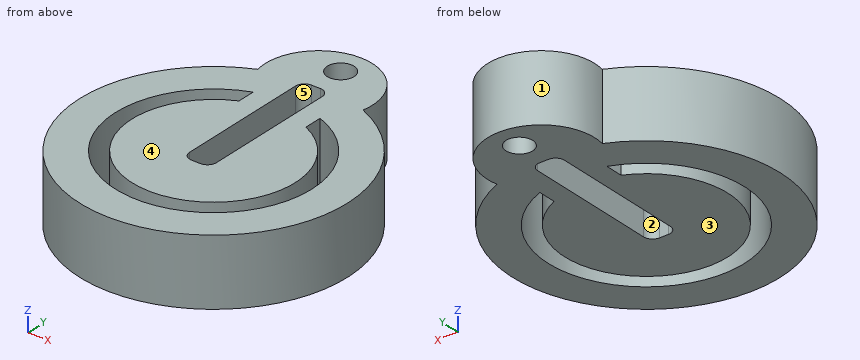
```python
from build123d import *

# Parameters (mm, degrees)
SKETCH_R     = 3
PAD_DEPTH    = 15
POCKET_DEPTH = 15.001


with BuildPart() as part:
    # Sketch → Pad (new body)
    with BuildSketch(Plane.XY):
        with BuildLine():
            ThreePointArc((-11.899095, 27.539273), (0.154021, -29.999605), (11.615696, 27.66))
            ThreePointArc((11.615696, 27.66), (-0.21563, 41.999446), (-11.899095, 27.539273))
        make_face()
        with Locations((0, 35.999605)):
            Circle(SKETCH_R, mode=Mode.SUBTRACT)
    extrude(amount=PAD_DEPTH)

    # Sketch001 (on Face5 of Pad) → Pocket (cut, through all)
    with BuildSketch(Plane.XY.offset(15)):
        with BuildLine():
            ThreePointArc((-7.5, 20.682118), (0, -22), (7.5, 20.682118))
            Line((7.5, 20.682118), (7.5, 16.682118))
            ThreePointArc((-7.5, 16.682118), (0, -18.290518), (7.5, 16.682118))
            Line((-7.5, 20.682118), (-7.5, 16.682118))
        make_face()
        with BuildLine():
            Line((-1, 29), (1, 29))
            ThreePointArc((3, 27), (2.414214, 28.414214), (1, 29))
            Line((3, 27), (3, -3))
            ThreePointArc((1, -5), (2.414214, -4.414214), (3, -3))
            Line((1, -5), (-1, -5))
            ThreePointArc((-3, -3), (-2.414214, -4.414214), (-1, -5))
            Line((-3, -3), (-3, 27))
            ThreePointArc((-1, 29), (-2.414214, 28.414214), (-3, 27))
        make_face()
    extrude(amount=-POCKET_DEPTH, mode=Mode.SUBTRACT)


solid = part.part
```
Work out the finished part from the listing and answer in its coordinate system (mm). Face numbers are marked on the shaded views. A direction names the side the tool comes from. Give positions to 0.01 mm unless a question says otherwise; leave off trailing zeros. Loops run counter-clockwise (first coordinate to the right, second up) from the corner with the lowest first, then second, coordinate; pieces in that order, holes last. Notation, with made-up numbers: (11, 42.5) - (27, 42.5) arc R12 ccw to (27, 64.5) - close; hole circle Ø7 at (73, 62.5). An arc over 180 degrees is marked (long way). One line per question, with ' | ' between items.
(1) The mould has two halves that part along X. Classify the marked faces 1, 2 and 3: +X half, -X half, draft (parallel to the pull), parting line (faces both ways), or undercut.
Recorded:
face 1: parting line | face 2: undercut | face 3: draft
(2) Each of these flat-tipped pins is pushed along its axis until it touches: pin 1 Ø4 at (x, y) = (-17.5, 28) entering from -Z; pin 2 Ø2 at (y, z) = (19, 11) entering from +X; pin 3 Ø1.5 at (x, z) = (10, 7.5) entering from +Y; pin 4 Ø1 at (y, z) = (-1, 12) entering from -X. Where does it stop, or does it pass through?
Recorded:
pin 1: passes through | pin 2: stops at x = 24 | pin 3: stops at y = 37.45 | pin 4: stops at x = -30
(3) The part is cut by section A-A (y = 0). Write down the section's boundary in (x, z), then the cut area to 3 significant figures.
Recorded:
outline: (-30, 0) - (-22, 0) - (-22, 15) - (-30, 15) - close; (-18.29, 0) - (-3, 0) - (-3, 15) - (-18.29, 15) - close; (3, 0) - (18.29, 0) - (18.29, 15) - (3, 15) - close; (22, 0) - (30, 0) - (30, 15) - (22, 15) - close | area: 699 mm²
(4) The part is cut by section B-B (x = -13.5). Write down the section's boundary in (y, z), then the cut area to 3 significant figures.
Recorded:
outline: (-26.79, 0) - (-17.37, 0) - (-17.37, 15) - (-26.79, 15) - close; (-12.34, 0) - (12.34, 0) - (12.34, 15) - (-12.34, 15) - close; (17.37, 0) - (26.79, 0) - (26.79, 15) - (17.37, 15) - close | area: 653 mm²
(5) A tool of negligible diameter and unlimited length cuts with its end or side. For the marked faces 4 and 5, from which of +Z, -Z, +X, -X, +Y, -Y can it reach the whole face along a straight path? Write none if from no direction.
Recorded:
face 4: +Z, +X, -X, +Y, -Y | face 5: +Z, -Z
(6) The part is cut by section C-C (z = 12.25). Write down the section's boundary in (x, y), then the cut area to 3 significant figures.
Recorded:
outline: (-11.9, 27.54) arc R30 ccw (long way) to (11.62, 27.66) arc R12 ccw (long way) to start; hole (-7.5, 16.68) - (-7.5, 20.68) arc R22 ccw (long way) to (7.5, 20.68) - (7.5, 16.68) arc R18.29 cw (long way) to start; hole (-3, -3) arc R2 ccw to (-1, -5) - (1, -5) arc R2 ccw to (3, -3) - (3, 27) arc R2 ccw to (1, 29) - (-1, 29) arc R2 ccw to (-3, 27) - close; hole circle Ø6 at (0, 36) | area: 2,430 mm²
(7) Straight lines are drawn through the part: probe 1 along X at (y, z) = (0, 6.5); probe 2 along Y at (x, z) = (-13.5, 0.75); probe 3 along X at (y, z) = (13, 3.75). For each, find the intervals that lie inside material, in ascending order.
Recorded:
probe 1: x = -30 to -22, -18.29 to -3, 3 to 18.29, 22 to 30 | probe 2: y = -26.79 to -17.37, -12.34 to 12.34, 17.37 to 26.79 | probe 3: x = -27.04 to -17.75, -12.87 to -3, 3 to 12.87, 17.75 to 27.04
(8) The part is cut by section D-D (x = 6.5). Write down the section's boundary in (y, z), then the cut area to 3 significant figures.
Recorded:
outline: (-29.29, 0) - (-21.02, 0) - (-21.02, 15) - (-29.29, 15) - close; (-17.1, 0) - (39.99, 0) - (39.99, 15) - (-17.1, 15) - close | area: 980 mm²
